Could you check a few things on this model? Use its own coordinates, in mm. Round coordinates to 2 decimals unless told otherwise and drop trailing zeros. Write each loop counter-clockwise with the first axis right and the second up, starting at its lowest first coordinate (ties: lowest second). Pieces come first, ordered by that corner, then holes. Notation, with made-up numbers: M -15,-32.5 L 6,-32.5 A27 ccw 6,-15.5 Z; hole C 73,58.5 d10. An arc over 180 degrees is marked long. One line per item, written item: value. Start each with the question number.
(1) I want a section at A-A on x = 16. Please give me the cut outline in (y, z).
(2) If I drill on L1, parallel to X at y = 21.5, z = 0.6; L2, parallel to Z at x = 12.75, y = 8.75; L3, parallel to Z at x = 25.5, y = 14.75, over which ranges is the centre line in solid material (lowest first)?
(3) I want a section at D-D on y = 24. Please give me the cut outline in (x, z), and give its area (3 significant figures).
(4) I want a section at B-B on z = 0.75. Please give me the cut outline in (x, y), and give its area (3 significant figures).
(5) I want a section at C-C on y = 15.25. Please give me the cut outline in (x, z).
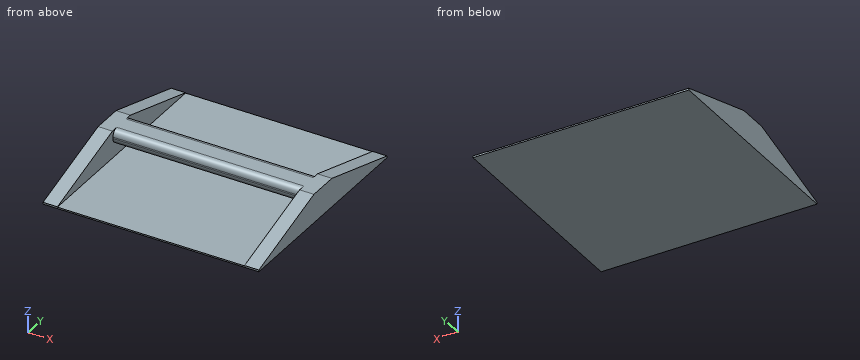
```python
from build123d import *

# Parameters (mm, degrees)
BOX001_W        = 2
BOX001_H        = 30
BOX001_DEPTH    = 4
BOX002_W        = 2
BOX002_H        = 30
BOX002_DEPTH    = 4
BOX003_W        = 26
BOX003_H        = 4
BOX003_DEPTH    = 2
FILLET_R        = 0.9
BOX_W           = 30
BOX_H           = 30
BOX_DEPTH       = 0.2
CHAMFER_1_SIZE2 = 3.75
CHAMFER_1_SIZE  = 12.9
CHAMFER_2_SIZE2 = 3.75
CHAMFER_2_SIZE  = 12.9
CHAMFER_3_SIZE2 = 12.9
CHAMFER_3_SIZE  = 3.75
CHAMFER_4_SIZE2 = 12.9
CHAMFER_4_SIZE  = 3.75


with BuildPart() as box001:
    # Box001 → Box001 (new body)
    with BuildSketch(Plane.XY):
        with Locations((1, 15)):
            Rectangle(BOX001_W, BOX001_H)
    extrude(amount=BOX001_DEPTH)


with BuildPart() as box002:
    # Box002 → Box002 (new body)
    with BuildSketch(Plane(origin=(28, 0, 0), x_dir=(1, 0, 0), z_dir=(0, 0, 1))):
        with Locations((1, 15)):
            Rectangle(BOX002_W, BOX002_H)
    extrude(amount=BOX002_DEPTH)


with BuildPart() as fillet_body:
    # Box003 → Box003 (new body)
    with BuildSketch(Plane(origin=(2, 13, 2), x_dir=(1, 0, 0), z_dir=(0, 0, 1))):
        with Locations((13, 2)):
            Rectangle(BOX003_W, BOX003_H)
    extrude(amount=BOX003_DEPTH)

    # Fillet
    fillet_edges = [fillet_body.edges().sort_by_distance(p)[0] for p in [
        (15, 13, 2),
        (15, 13, 4),
        (15, 17, 2),
        (15, 17, 4),
    ]]
    fillet(fillet_edges, radius=FILLET_R)


with BuildPart() as strapassembly:
    # Box → Box (new body)
    with BuildSketch(Plane.XY):
        with Locations((15, 15)):
            Rectangle(BOX_W, BOX_H)
    extrude(amount=BOX_DEPTH)

    # Fusion: union Box001, Box002, Fillet body
    add(box001.part)
    add(box002.part)
    add(fillet_body.part)

    # Chamfer 1
    chamfer_1_edges = [strapassembly.edges().sort_by_distance(p)[0] for p in [
        (29, 30, 4),
    ]]
    chamfer_1_side = strapassembly.faces().sort_by_distance((29, 15, 4))[0]
    chamfer(chamfer_1_edges, length=CHAMFER_1_SIZE, length2=CHAMFER_1_SIZE2, reference=chamfer_1_side)

    # Chamfer 2
    chamfer_2_edges = [strapassembly.edges().sort_by_distance(p)[0] for p in [
        (1, 30, 4),
    ]]
    chamfer_2_side = strapassembly.faces().sort_by_distance((1, 15, 4))[0]
    chamfer(chamfer_2_edges, length=CHAMFER_2_SIZE, length2=CHAMFER_2_SIZE2, reference=chamfer_2_side)

    # Chamfer 3
    chamfer_3_edges = [strapassembly.edges().sort_by_distance(p)[0] for p in [
        (29, 0, 4),
    ]]
    chamfer_3_side = strapassembly.faces().sort_by_distance((29, 0, 2.1))[0]
    chamfer(chamfer_3_edges, length=CHAMFER_3_SIZE, length2=CHAMFER_3_SIZE2, reference=chamfer_3_side)

    # Chamfer 4
    chamfer_4_edges = [strapassembly.edges().sort_by_distance(p)[0] for p in [
        (1, 0, 4),
    ]]
    chamfer_4_side = strapassembly.faces().sort_by_distance((1, 0, 2.1))[0]
    chamfer(chamfer_4_edges, length=CHAMFER_4_SIZE, length2=CHAMFER_4_SIZE2, reference=chamfer_4_side)


solid = strapassembly.part
```
Found:
1. outline: M 0,0 L 30,0 L 30,0.2 L 0,0.2 Z; M 13,2.9 A0.9 ccw 13.9,2 L 16.1,2 A0.9 ccw 17,2.9 L 17,3.1 A0.9 ccw 16.1,4 L 13.9,4 A0.9 ccw 13,3.1 Z
2. L1: x = 0 to 2, 28 to 30
2. L2: z = 0 to 0.2
2. L3: z = 0 to 0.2, 2 to 4
3. outline: M 0,0 L 30,0 L 30,1.99 L 28,1.99 L 28,0.2 L 2,0.2 L 2,1.99 L 0,1.99 Z
3. area: 13.2 mm²
4. outline: M 0,1.72 L 2,1.72 L 2,28.28 L 0,28.28 Z; M 28,1.72 L 30,1.72 L 30,28.28 L 28,28.28 Z
4. area: 106 mm²
5. outline: M 0,0 L 30,0 L 30,4 L 0,4 Z; hole M 2,0.2 L 28,0.2 L 28,2 L 2,2 Z
